Verification items for the finished model (mm, model axes). Round coordinates to 2 decimals unless told otherwise and drop trailing zeros. Loops run counter-clockwise (first coordinate to the right, second up) from the corner with the lowest first, then second, coordinate; pieces in that order, holes last. Notation, with made-up numbers: M 8,-7.75 L 24,-7.75 A23 ccw 24,0.25 Z; hole C 76,27 d3. An arc over 180 degrees is marked long. One line per item, written item: value.
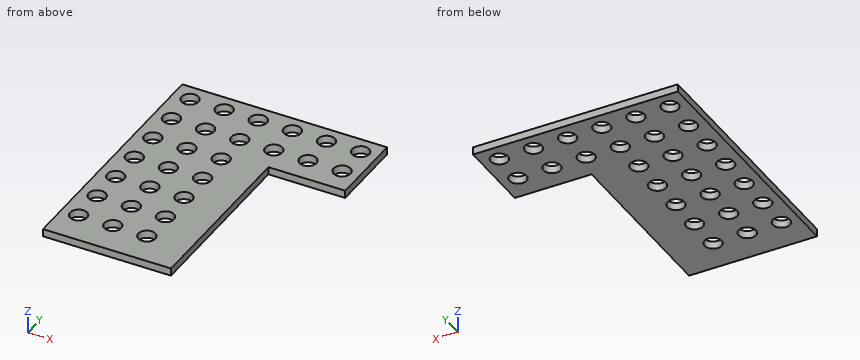
from build123d import *

# Parameters (mm, degrees)
BOSS_EXTRUDE1_DEPTH     = 4.5
SKETCH3_R               = 5
CUT_EXTRUDE1_DEPTH      = 97.152223063
FILL_PATTERN1_OUTLINE_R = 5
FILL_PATTERN1_DEPTH     = 4.5


# Read off the part's stored shape, not the designer's step: Fill Pattern1
with BuildPart() as part:
    # Sketch2 → Boss-Extrude1 (new body)
    with BuildSketch(Plane.XY):
        Polygon((15, -75), (-60, -75), (-60, 75), (60, 75), (60, 30), (15, 30), align=None)
    extrude(amount=BOSS_EXTRUDE1_DEPTH)

    # Sketch3 → Cut-Extrude1 (cut, through all)
    with BuildSketch(Plane.XY.offset(4.5)):
        with Locations((-50, 65)):
            Circle(SKETCH3_R)
    extrude(amount=-CUT_EXTRUDE1_DEPTH, mode=Mode.SUBTRACT)

    # Fill Pattern1 outline → Fill Pattern1 (cut)
    with BuildSketch(Plane.XY):
        with Locations((-30, 65)):
            Circle(FILL_PATTERN1_OUTLINE_R)
        with Locations((-30, -55)):
            Circle(FILL_PATTERN1_OUTLINE_R)
        with Locations((-10, -55)):
            Circle(FILL_PATTERN1_OUTLINE_R)
        with Locations((-50, -35)):
            Circle(FILL_PATTERN1_OUTLINE_R)
        with Locations((-30, -35)):
            Circle(FILL_PATTERN1_OUTLINE_R)
        with Locations((-50, -15)):
            Circle(FILL_PATTERN1_OUTLINE_R)
        with Locations((50, 65)):
            Circle(FILL_PATTERN1_OUTLINE_R)
        with Locations((50, 45)):
            Circle(FILL_PATTERN1_OUTLINE_R)
        with Locations((-10, -35)):
            Circle(FILL_PATTERN1_OUTLINE_R)
        with Locations((-50, -55)):
            Circle(FILL_PATTERN1_OUTLINE_R)
        with Locations((-10, 25)):
            Circle(FILL_PATTERN1_OUTLINE_R)
        with Locations((-30, 25)):
            Circle(FILL_PATTERN1_OUTLINE_R)
        with Locations((-50, 25)):
            Circle(FILL_PATTERN1_OUTLINE_R)
        with Locations((10, 65)):
            Circle(FILL_PATTERN1_OUTLINE_R)
        with Locations((-10, 45)):
            Circle(FILL_PATTERN1_OUTLINE_R)
        with Locations((-10, 65)):
            Circle(FILL_PATTERN1_OUTLINE_R)
        with Locations((-50, 45)):
            Circle(FILL_PATTERN1_OUTLINE_R)
        with Locations((-30, 45)):
            Circle(FILL_PATTERN1_OUTLINE_R)
        with Locations((-30, -15)):
            Circle(FILL_PATTERN1_OUTLINE_R)
        with Locations((-10, -15)):
            Circle(FILL_PATTERN1_OUTLINE_R)
        with Locations((30, 45)):
            Circle(FILL_PATTERN1_OUTLINE_R)
        with Locations((30, 65)):
            Circle(FILL_PATTERN1_OUTLINE_R)
        with Locations((-50, 5)):
            Circle(FILL_PATTERN1_OUTLINE_R)
        with Locations((-30, 5)):
            Circle(FILL_PATTERN1_OUTLINE_R)
        with Locations((-10, 5)):
            Circle(FILL_PATTERN1_OUTLINE_R)
        with Locations((10, 45)):
            Circle(FILL_PATTERN1_OUTLINE_R)
    extrude(amount=FILL_PATTERN1_DEPTH, mode=Mode.SUBTRACT)


solid = part.part
(1) Thickness scan on L1, parallel to X at y = -35.5, z = 3.35; L2, parallel to Y at x = 50, z = 2.7; L3, parallel to Y at x = 26, z = 0.85. Record the ranges inside material, lowest first. Write a range as from..to.
Completed:
L1: x = -60..-54.97, -45.03..-34.97, -25.03..-14.97, -5.03..15
L2: y = 30..40, 50..60, 70..75
L3: y = 30..42, 48..62, 68..75
(2) Sectioned sample at C-C on z = 2.3. Count the separate pieces of the cut face and the enclosed holes in it, and give its area (3 significant figures).
Completed:
separate pieces: 1
enclosed holes: 27
area: 11,200 mm^2
(3) Sectioned sample at A-A on y = -55. Enter the section's corners in (x, z).
Completed:
outline: M -60,0 L -55,0 L -55,4.5 L -60,4.5 Z; M -45,0 L -35,0 L -35,4.5 L -45,4.5 Z; M -25,0 L -15,0 L -15,4.5 L -25,4.5 Z; M -5,0 L 15,0 L 15,4.5 L -5,4.5 Z
(4) Sectioned sample at B-B on x = 47. Enter the section's corners in (y, z).
Completed:
outline: M 30,0 L 41,0 L 41,4.5 L 30,4.5 Z; M 49,0 L 61,0 L 61,4.5 L 49,4.5 Z; M 69,0 L 75,0 L 75,4.5 L 69,4.5 Z
